Autodesk Inventor part; units mm, degrees
ref_plane "YZ Plane" through (0, 0, 0) normal (1, 0, 0) x (0, 1, 0)
ref_plane "XZ Plane" through (0, 0, 0) normal (0, 1, 0) x (-1, 0, 0)
ref_plane "XY Plane" through (0, 0, 0) normal (0, 0, 1) x (1, 0, 0)
sketch "Sketch1" plane through (0, 0, 0) normal (1, 0, 0) x (0, 1, 0)
  line L0 (0, 9.5) -> (0, -9.5)
  line L1 (0, -9.5) -> (8, -9.5)
  line L2 (0, 9.5) -> (8, 9.5)
  line L3 (8, 9.5) -> (8, 14.5)
  line L4 (8, 14.5) -> (9.5, 14.5)
  line L5 (9.5, 14.5) -> (9.5, 10.5)
  line L6 (9.5, 10.5) -> (11.5, 10.5)
  line L7 (11.5, 10.5) -> (11.5, 16.5)
  line L8 (11.5, 16.5) -> (6, 16.5)
  line L9 (6, 16.5) -> (6, 11.5)
  line L10 (6, 11.5) -> (-3, 11.5)
  line L11 (-3, 11.5) -> (-4, 11.5)
  line L12 (-4, 11.5) -> (-4, 1)
  line L13 (0, 0) -> (3.5, 0)
  line L14 (0, -9.5) -> (8, -9.5)
  line L15 (8, -9.5) -> (8, -14.5)
  line L16 (8, -14.5) -> (9.5, -14.5)
  line L17 (9.5, -14.5) -> (9.5, -10.5)
  line L18 (11.5, -10.5) -> (11.5, -16.5)
  line L19 (11.5, -16.5) -> (6, -16.5)
  line L20 (6, -16.5) -> (6, -11.5)
  line L21 (6, -11.5) -> (-3, -11.5)
  line L22 (-3, -11.5) -> (-4, -11.5)
  line L23 (-4, -11.5) -> (-4, 1)
  line L24 (11.5, -10.5) -> (9.5, -10.5)
  point P0 (8.75, -16.5)
  point P1 (8.75, -14.5)
  dimension "d0" = 19
  dimension "d1" = 0
  dimension "d2" = 8
  dimension "d3" = 8
  dimension "d4" = 5
  dimension "d5" = 1.5
  dimension "d6" = 2
  dimension "d7" = 6
  dimension "d8" = 5.5
  dimension "d9" = 5
  dimension "d10" = 1
  dimension "d13" = 2
  dimension "d14" = 4
extrude "Extrusion1" add sketch "Sketch1" along normal blind 20
fillet "Fillet1" radius 5 2 edges at (10, 6, -11.5) (10, 6, 11.5)
chamfer "Chamfer1" distance 1 angle 45 12 edges at (20, 8, -12) (20, 8.75, -14.5) (20, 9.5, -12.5) (20, 8, 12) (20, 8.75, 14.5) (20, 9.5, 12.5) (0, 8, -12) (0, 8.75, -14.5) (0, 9.5, -12.5) (0, 8, 12) (0, 8.75, 14.5) (0, 9.5, 12.5)
sketch "Sketch3" plane through (0, -4, -11.5) normal (0, -1, 0) x (1, 0, 0)
  line L0 (6, 15.5002) -> (13.9, 15.5002)
  line L1 (13.9, 15.5002) -> (13.9, 7.6002)
  line L2 (13.9, 7.6002) -> (6, 7.6002)
  line L3 (6, 7.6002) -> (6, 15.5002)
  line L4 (0, 23) -> (0, 0)
  line L5 (0, 23) -> (20, 23)
  point P0 (0, 11.5)
  point P1 (10, 23)
  point P2 (9.95, 15.5002)
  dimension "d27" = 7.9
  dimension "d28" = 7.9
  dimension "d29" = 6
  dimension "d30" = 7.5
extrude "Extrusion3" add sketch "Sketch3" along normal blind 2.49
sketch "Sketch4" plane through (0, -6.49, -11.5) normal (0, -1, 0) x (1, 0, 0)
  line L0 (1.5, 15.5002) -> (18.4, 15.5002)
  line L1 (18.4, 15.5002) -> (18.4, 7.6002)
  line L2 (18.4, 7.6002) -> (1.5, 7.6002)
  line L3 (1.5, 7.6002) -> (1.5, 15.5002)
  line L4 (1.5, 15.5002) -> (18.4, 7.6002) construction
  line L5 (18.4, 15.5002) -> (1.5, 7.6002) construction
  line L6 (6, 7.6002) -> (13.9, 7.6002)
  line L7 (13.9, 7.6002) -> (13.9, 15.5002)
  point P0 (0, 11.5)
  point P1 (9.95, 11.5502)
  dimension "d33" = 16.9
  dimension "d34" = 7.9
  dimension "d35" = 0
  dimension "d36" = 4.5
extrude "Extrusion4" add sketch "Sketch4" along normal blind 3
fillet "Fillet2" radius 5 4 edges at (6, -5.245, -3.8998) (1.5, -7.99, -3.8998) (13.9, -5.245, 4.0002) (18.4, -7.99, 4.0002)
sketch "Sketch2" plane through (0, 0, 9.5) normal (0, 1, 0) x (1, 0, 0)
  circle A0 centre (10, 9.5) radius 3
  line L0 (20, 19) -> (20, 0)
  line L1 (0, -7) -> (20, -7)
  point P0 (0, 9.5)
  dimension "d19" = 6
  dimension "d20" = 10
  dimension "d21" = 16.5
properties part number "Drziak_3"
Check sheet for the modelled part. Datum: model origin and axes. Units: mm. A direction names the side the tool comes from. Coordinates: 2 decimals unless noted, no trailing zeros. Loops run counter-clockwise (first coordinate to the right, second up) from the corner with the lowest first, then second, coordinate; pieces in that order, holes last.
1) Release check for a two-part mould opening along Z. For faces 1 (the face through (19.6, 8.7, 15.1)), 2 (the face through (10, 9, 16.5)), 3 (the face through (19.5, 10, -13)), 4 (the face through (10, 9, -16.5)) record: released by +Z, released by -Z, zero draft, split by the parting line, or undercut.
2) Sectioned sample at C-C (y = 4). Record the boundary of the cut face in (x, z).
3) Sectioned sample at B-B (z = -13.5). Record the boundary of the cut face in (x, y).
4) Sectioned sample at D-D (y = -8). Record the boundary of the cut face in (x, z).
5) Access from +Z, -Z, +X, -X, +Y, -Y to the whole of each face (thin tool, end or side, straight path). Record for faces 5 (the face through (0.5, 7.5, -12.5)), 6 (the face through (10, 4, -9.5)), 7 (the face through (10, -1, 11.5)), 8 (the face through (10, 8, 12)).
6) Material ranges on probe 1 along Z at (x, y) = (6.75, 10.5); probe 2 along Y at (x, z) = (17, 12.5); probe 3 along Z at (x, y) = (13, 6.25), recorded low to high.
7) Gauge pin test, flat ends, axial feed: pin 1 (2.5 mm diameter, centred on x = 13, y = -7, fed in from -Z); pin 2 (6.5 mm diameter, centred on x = 15, z = 0.5, fed in from +Y); pin 3 (4 mm diameter, centred on x = 6.5, y = -1, fed in from +Z). Record the tip position at first contact, or that the pin passes through.
Check sheet entries:
1. face 1: undercut
1. face 2: released by +Z
1. face 3: undercut
1. face 4: released by -Z
2. outline: (0, -12.5) - (20, -12.5) - (20, -9.5) - (0, -9.5) - close; (0, 9.5) - (20, 9.5) - (20, 12.5) - (0, 12.5) - close
3. outline: (0, 5) - (20, 5) - (20, 7) - (19, 8) - (1, 8) - (0, 7) - close; (0, 10.5) - (1, 9.5) - (19, 9.5) - (20, 10.5) - (20, 11.5) - (0, 11.5) - close
4. outline: (1.5, 1.1) arc R5 ccw to (6.5, -3.9) - (18.4, -3.9) - (18.4, -1) arc R5 ccw to (13.4, 4) - (1.5, 4) - close
5. face 5: -X
5. face 6: +X, -X, +Y
5. face 7: +Z, +X, -X, -Y
5. face 8: +X, -X
6. probe 1: z = -16.5 to -10.5, 10.5 to 16.5
6. probe 2: y = 4 to 8, 9.5 to 11.5
6. probe 3: z = -16.5 to -9.5, 9.5 to 16.5
7. pin 1: stops at z = -3.9
7. pin 2: stops at y = 0
7. pin 3: stops at z = 11.5
